Can you work these out from the model? Positions are in its coordinate system, mm. Face numbers are marked on the shaded views. A direction names the side the tool comes from. Round coordinates to 2 decimals unless told otherwise and drop trailing zeros. Loops run counter-clockwise (first coordinate to the right, second up) from the corner with the lowest first, then second, coordinate; pieces in that order, holes last.
from build123d import *

# Parameters (mm, degrees)
SKETCH_1_W                = 40
SKETCH_1_H                = 40
EXTRUDE_1_DEPTH           = 5
SKETCH_2_R                = 1.5
SKETCH_2_R_2              = 16
CUT_EXTRUDE_1_DEPTH       = 29.722813233
SKETCH_3_W                = 6
SKETCH_3_H                = 5
EXTRUDE_2_DEPTH           = 10
SKETCH_4_R                = 3
EXTRUDE_3_DEPTH           = 6
EXTRUDE_START             = -6
SKETCH_5_R                = 3
EXTRUDE_4_DEPTH           = 6
CUT_EXTRUDE_2_DEPTH       = 44.488504228
SKETCH_7_R                = 1.5
CUT_EXTRUDE_3_DEPTH       = 43.133715716
SKETCH_9_R                = 4
EXTRUDE_5_DEPTH           = 6
SKETCH_10_R               = 4
EXTRUDE_6_DEPTH           = 6
SKETCH_11_R               = 1.5
CUT_EXTRUDE_4_DEPTH       = 43.944731924
CUT_EXTRUDE_5_DEPTH       = 13
CUT_EXTRUDE_5_DEPTH_BACK  = 3
FILLET_1_R                = 3
CUT_EXTRUDE_6_DEPTH       = 3
CUT_EXTRUDE_7_DEPTH       = 3
SKETCH_15_R               = 1.65
CUT_EXTRUDE_8_DEPTH       = 43.944731924
SKETCH_16_R               = 5
EXTRUDE_7_DEPTH           = 6
SKETCH_17_R               = 5
EXTRUDE_8_DEPTH           = 6
SKETCH_18_R               = 1.7
CUT_EXTRUDE_9_DEPTH       = 44.786413418
CUT_EXTRUDE_10_DEPTH      = 13
CUT_EXTRUDE_10_DEPTH_BACK = 3
SKETCH_20_R               = 17.5
CUT_EXTRUDE_11_DEPTH      = 37.827299657


with BuildPart() as part:
    # Эскиз1 → Бобышка-Вытянуть1 (new body)
    with BuildSketch(Plane.XY):
        Rectangle(SKETCH_1_W, SKETCH_1_H)
    extrude(amount=EXTRUDE_1_DEPTH)

    # Эскиз2 → Вырез-Вытянуть1 (cut, through all)
    with BuildSketch(Plane.XY.offset(5)):
        with Locations((-16, 16)):
            Circle(SKETCH_2_R)
        Circle(SKETCH_2_R_2)
        with Locations((16, 16)):
            Circle(SKETCH_2_R)
        with Locations((16, -16)):
            Circle(SKETCH_2_R)
        with Locations((-16, -16)):
            Circle(SKETCH_2_R)
    extrude(amount=-CUT_EXTRUDE_1_DEPTH, mode=Mode.SUBTRACT)

    # Эскиз3 → Бобышка-Вытянуть2 (add)
    with BuildSketch(Plane(origin=(0, 20, 0), x_dir=(1, 0, 0), z_dir=(0, 1, 0))):
        with Locations((-8, -2.5)):
            Rectangle(SKETCH_3_W, SKETCH_3_H)
        with Locations((8, -2.5)):
            Rectangle(SKETCH_3_W, SKETCH_3_H)
    extrude(amount=EXTRUDE_2_DEPTH)

    # Эскиз4 → Бобышка-Вытянуть3 (add)
    with BuildSketch(Plane.ZY.offset(11)):
        with Locations((2.5, 25)):
            Circle(SKETCH_4_R)
    extrude(amount=-EXTRUDE_3_DEPTH)

    # Эскиз5 → Бобышка-Вытянуть4 (add)
    with BuildSketch(Plane(origin=(11, 0, 0), x_dir=(0, 0, -1), z_dir=(1, 0, 0)).offset(EXTRUDE_START)):
        with Locations((-2.5, 25)):
            Circle(SKETCH_5_R)
    extrude(amount=EXTRUDE_4_DEPTH)

    # Эскиз6 → Вырез-Вытянуть2 (cut, through all)
    with BuildSketch(Plane(origin=(11, 0, 0), x_dir=(0, 0, -1), z_dir=(1, 0, 0))):
        with BuildLine():
            Line((0, 30), (-5, 30))
            Line((-5, 30), (-5, 26.658312395))
            ThreePointArc((-5, 26.658312395), (-2.5, 28), (0, 26.658312395))
            Line((0, 26.658312395), (0, 30))
        make_face()
    extrude(amount=-CUT_EXTRUDE_2_DEPTH, mode=Mode.SUBTRACT)

    # Эскиз7 → Вырез-Вытянуть3 (cut, through all)
    with BuildSketch(Plane.ZY.offset(11)):
        with Locations((2.5, 25)):
            Circle(SKETCH_7_R)
    extrude(amount=-CUT_EXTRUDE_3_DEPTH, mode=Mode.SUBTRACT)

    # Эскиз9 → Бобышка-Вытянуть5 (add)
    with BuildSketch(Plane.ZY.offset(11)):
        with Locations((2.5, 25)):
            Circle(SKETCH_9_R)
    extrude(amount=-EXTRUDE_5_DEPTH)

    # Эскиз10 → Бобышка-Вытянуть6 (add)
    with BuildSketch(Plane(origin=(11, 0, 0), x_dir=(0, 0, -1), z_dir=(1, 0, 0)).offset(EXTRUDE_START)):
        with Locations((-2.5, 25)):
            Circle(SKETCH_10_R)
    extrude(amount=EXTRUDE_6_DEPTH)

    # Эскиз11 → Вырез-Вытянуть4 (cut, through all)
    with BuildSketch(Plane(origin=(11, 0, 0), x_dir=(0, 0, -1), z_dir=(1, 0, 0))):
        with Locations((-2.5, 25)):
            Circle(SKETCH_11_R)
    extrude(amount=-CUT_EXTRUDE_4_DEPTH, mode=Mode.SUBTRACT)

    # Эскиз12 → Вырез-Вытянуть5 (cut, two sides: drawn at the far end of the back side and taken through both)
    with BuildSketch(Plane(origin=(-5, 0, 0), x_dir=(0, 0, -1), z_dir=(1, 0, 0)).offset(-CUT_EXTRUDE_5_DEPTH_BACK)):
        Polygon((-0.91228676, 22.25), (0.675426481, 25), (-0.91228676, 27.75), (-4.08771324, 27.75), (-5.675426481, 25), (-4.08771324, 22.25), align=None)
    extrude(amount=CUT_EXTRUDE_5_DEPTH + CUT_EXTRUDE_5_DEPTH_BACK, mode=Mode.SUBTRACT)

    # Скругление1
    fillet_1_edges = [part.edges().sort_by_distance(p)[0] for p in [
        (20, -20, 2.5),
        (-20, -20, 2.5),
        (-20, 20, 2.5),
        (20, 20, 2.5),
    ]]
    fillet(fillet_1_edges, radius=FILLET_1_R)

    # Эскиз13 → Вырез-Вытянуть6 (cut)
    with BuildSketch(Plane(origin=(-5, 0, 0), x_dir=(0, 0, -1), z_dir=(1, 0, 0))):
        Polygon((-4.174315781, 22.1), (-0.825684219, 22.1), (0.848631561, 25), (-0.825684219, 27.9), (-4.174315781, 27.9), (-5.848631561, 25), align=None)
    extrude(amount=-CUT_EXTRUDE_6_DEPTH, mode=Mode.SUBTRACT)

    # Эскиз14 → Вырез-Вытянуть7 (cut)
    with BuildSketch(Plane.ZY.offset(-5)):
        Polygon((4.174315781, 22.1), (5.848631561, 25), (4.174315781, 27.9), (0.825684219, 27.9), (-0.848631561, 25), (0.825684219, 22.1), align=None)
    extrude(amount=-CUT_EXTRUDE_7_DEPTH, mode=Mode.SUBTRACT)

    # Эскиз15 → Вырез-Вытянуть8 (cut, through all)
    with BuildSketch(Plane.ZY.offset(11)):
        with Locations(Location((2.5, 25, 0), (0, 0, 180))):
            Circle(SKETCH_15_R)
    extrude(amount=-CUT_EXTRUDE_8_DEPTH, mode=Mode.SUBTRACT)

    # Эскиз16 → Бобышка-Вытянуть7 (add)
    with BuildSketch(Plane.ZY.offset(11)):
        with Locations((2.5, 25)):
            Circle(SKETCH_16_R)
    extrude(amount=-EXTRUDE_7_DEPTH)

    # Эскиз17 → Бобышка-Вытянуть8 (add)
    with BuildSketch(Plane(origin=(11, 0, 0), x_dir=(0, 0, -1), z_dir=(1, 0, 0)).offset(EXTRUDE_START)):
        with Locations((-2.5, 25)):
            Circle(SKETCH_17_R)
    extrude(amount=EXTRUDE_8_DEPTH)

    # Эскиз18 → Вырез-Вытянуть9 (cut, through all)
    with BuildSketch(Plane(origin=(11, 0, 0), x_dir=(0, 0, -1), z_dir=(1, 0, 0))):
        with Locations((-2.5, 25)):
            Circle(SKETCH_18_R)
    extrude(amount=-CUT_EXTRUDE_9_DEPTH, mode=Mode.SUBTRACT)

    # Эскиз19 → Вырез-Вытянуть10 (cut, two sides: drawn at the far end of the back side and taken through both)
    with BuildSketch(Plane(origin=(-5, 0, 0), x_dir=(0, 0, -1), z_dir=(1, 0, 0)).offset(-CUT_EXTRUDE_10_DEPTH_BACK)):
        Polygon((-4.203183294, 22.05), (-0.796816706, 22.05), (0.906366588, 25), (-0.796816706, 27.95), (-4.203183294, 27.95), (-5.906366588, 25), align=None)
    extrude(amount=CUT_EXTRUDE_10_DEPTH + CUT_EXTRUDE_10_DEPTH_BACK, mode=Mode.SUBTRACT)

    # Эскиз20 → Вырез-Вытянуть11 (cut, through all)
    with BuildSketch(Plane.XY.offset(5)):
        Circle(SKETCH_20_R)
    extrude(amount=-CUT_EXTRUDE_11_DEPTH, mode=Mode.SUBTRACT)


solid = part.part
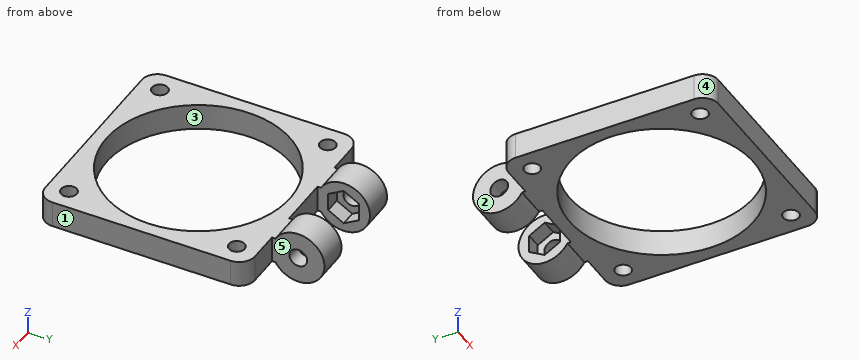
(1) If I drill on line 1 (Y direction, x = 0, z = 2.25); line 2 (Y direction, x = -16, z = 3.8); line 3 (X direction, y = -15.5, z = 0.5), over which ranges is the centre line in solid material (lowest first)?
Worked answers:
line 1: y = -20 to -17.5, 17.5 to 20
line 2: y = -20 to -17.5, -14.5 to -7.09, 7.09 to 14.5, 17.5 to 20
line 3: x = -20 to -17.41, -14.59 to -8.12, 8.12 to 14.59, 17.41 to 20
(2) If we section it at D-D, the plane y = 6: List the corners of the cut face in (x, z) for me, then the cut area to 3 significant figures.
Worked answers:
outline: (-20, 0) - (-16.44, 0) - (-16.44, 5) - (-20, 5) - close; (16.44, 0) - (20, 0) - (20, 5) - (16.44, 5) - close
area: 35.6 mm2
(3) For the marked faces 4 and 5, which set-ups out of +Z, -Z, +X, -X, +Y, -Y let a thin tool reach every point of the face, with its end or its side?
Worked answers:
face 4: +Z, -Z, -X, -Y
face 5: +Z, -Z, +X, +Y
(4) If we section it at A-A, the plane y = 26: List the corners of the cut face in (x, z) for me.
Worked answers:
outline: (-11, -2.4) - (-5, -2.4) - (-5, -0.33) - (-8, -0.33) - (-8, 1.13) - (-11, 1.13) - close; (-11, 3.87) - (-8, 3.87) - (-8, 5.33) - (-5, 5.33) - (-5, 7.4) - (-11, 7.4) - close; (5, -2.4) - (11, -2.4) - (11, 1.13) - (8, 1.13) - (8, -0.33) - (5, -0.33) - close; (5, 5.33) - (8, 5.33) - (8, 3.87) - (11, 3.87) - (11, 7.4) - (5, 7.4) - close
(5) If we section it at C-C, the plane z = 2.5: State how many separate pieces and enclosed holes the cut face has, then the cut area to 3 significant figures.
Worked answers:
separate pieces: 3
enclosed holes: 5
area: 666 mm2
(6) If we mould it in two halves opening along X, with no side actions, what happens to the marked faces 1, 2 and 3? For each: released by +X, released by -X, zero draft, split by the parting line, or undercut.
Worked answers:
face 1: released by +X
face 2: released by -X
face 3: undercut
(7) Will these pins go through, and if not, where does the flat tip stop? P1, Ø3, axis at y = 24.5, z = 1.5, coming from the -X side; P2, Ø20, axis at x = 2.5, y = 0.5, coming from the -Z side; P3, Ø2.5, axis at x = -15.5, z = 2.5, coming from the +Y side; P4, Ø5, axis at x = 11.5, y = -14, coming from the +Z side.
Worked answers:
P1: stops at x = -11
P2: passes through
P3: stops at y = 20
P4: stops at z = 5
(8) If we section it at B-B, the plane x = 16: List the corners of the cut face in (y, z) for me.
Worked answers:
outline: (-20, 0) - (-17.5, 0) - (-17.5, 5) - (-20, 5) - close; (-14.5, 0) - (-7.09, 0) - (-7.09, 5) - (-14.5, 5) - close; (7.09, 0) - (14.5, 0) - (14.5, 5) - (7.09, 5) - close; (17.5, 0) - (20, 0) - (20, 5) - (17.5, 5) - close
